Could you check a few things on this model? Use its own coordinates, in mm. A direction names the side the tool comes from. Give positions to 0.01 mm unless a question says otherwise; leave off trailing zeros. Write each loop counter-clockwise with the first axis right and the second up, starting at its lowest first coordinate (ties: lowest second). Pieces come first, ordered by that corner, then holes. Notation, with made-up numbers: (44.5, -26.75) - (49.5, -26.75) arc R11 cw to (49.5, -11.75) - close; hole circle Ø9 at (16, 63). An arc over 180 degrees is marked (long way). Answer in a Markdown table with one row per item.
from build123d import *

# Parameters (mm, degrees)
BOSS_EXTRUDE1_DEPTH = 300


with BuildPart() as part:
    # Sketch3 → Boss-Extrude1 (new body)
    with BuildSketch(Plane.XY):
        with BuildLine():
            Line((-25, 0), (25, 0))
            Line((25, 0), (25, 17.5))
            ThreePointArc((25, 17.5), (23.535533906, 21.035533906), (20, 22.5))
            Line((20, 22.5), (16.770509831, 22.5))
            ThreePointArc((16.770509831, 22.5), (13.782438308, 21.508918629), (11.978935594, 18.928571429))
            ThreePointArc((11.978935594, 18.928571429), (0, 10), (-11.978935594, 18.928571429))
            ThreePointArc((-11.978935594, 18.928571429), (-13.782438308, 21.508918629), (-16.770509831, 22.5))
            Line((-16.770509831, 22.5), (-20, 22.5))
            ThreePointArc((-20, 22.5), (-23.535533906, 21.035533906), (-25, 17.5))
            Line((-25, 17.5), (-25, 0))
        make_face()
    extrude(amount=BOSS_EXTRUDE1_DEPTH)


solid = part.part
1) On a 3-axis mill with a long thin cutter (end or side, diameter ignored), from which of +Z, -Z, +X, -X, +Y, -Y can I reach the whole of each face in a straight line? I mean faces 1 (the face through (13.819, 21.536, 147.9)), 2 (the face through (0, 0, 148)). Say none if no direction works.
Check values:
| item | result |
|---|---|
| face 1 | +Z, -Z, +Y |
| face 2 | +Z, -Z, +X, -X, -Y |
2) If I drill on line 1 (Y direction, x = 16, z = 208.5); line 2 (X direction, y = 18.25, z = 34); line 3 (X direction, y = 17, z = 274.5), over which ranges is the centre line in solid material (lowest first)?
Check values:
| item | result |
|---|---|
| line 1 | y = 0 to 22.44 |
| line 2 | x = -24.94 to -11.76, 11.76 to 24.94 |
| line 3 | x = -25 to -11.22, 11.22 to 25 |
3) We'd pull the mould along X, two halves only. Please class faces 3 (the face through (0, 9, 300)), 4 (the face through (0, 10, 148)), 5 (the face through (23.57, 21, 147.9)): +X half, -X half, draft (parallel to the pull), parting line (faces both ways), or undercut.
Check values:
| item | result |
|---|---|
| face 3 | draft |
| face 4 | undercut |
| face 5 | +X half |
4) Will this pin go through, and if not, where does the flat tip stop? P1, Ø5, axis at x = 2.5, z = 125, coming from the +Y side.
Check values:
| item | result |
|---|---|
| P1 | stops at y = 11.04 |
5) Imagine slicing it at B-B (x = -0.5). List the corners of the cut face in (y, z) for me.
Check values:
| item | result |
|---|---|
| outline | (0, 0) - (10.01, 0) - (10.01, 300) - (0, 300) - close |
6) Imagine slicing it at A-A (z = 19.5). List the corners of the cut face in (x, y) for me, then the cut area to 3 significant figures.
Check values:
| item | result |
|---|---|
| outline | (-25, 0) - (25, 0) - (25, 17.5) arc R5 ccw to (20, 22.5) - (16.77, 22.5) arc R5 ccw to (11.98, 18.93) arc R12.5 cw to (-11.98, 18.93) arc R5 ccw to (-16.77, 22.5) - (-20, 22.5) arc R5 ccw to (-25, 17.5) - close |
| area | 862 mm2 |
